Could you check a few things on this model? Use its own coordinates, in mm. A direction names the side the tool comes from. Coordinates: 2 decimals unless noted, no trailing zeros. Loops run counter-clockwise (first coordinate to the right, second up) from the corner with the lowest first, then second, coordinate; pieces in that order, holes last. Notation, with made-up numbers: (-24, 55.25) - (34, 55.25) arc R26 ccw to (34, 78.25) - close; hole circle Ø5 at (-9.5, 23.5). An arc over 180 degrees is marked (long way). One line per question, with ' | ' between items. Start each with the question number.
1. Which directions (+Z, -Z, +X, -X, +Y, -Y) give clear straight access to the entire face, cutting with the end or side of a thin tool? Please do faces 1 (the cylindrical face through (-0.116, -88.438, 49.823)), 2 (the flat face through (1.412, -89, 14)), 3 (the flat face through (-17, -89, -24.929)).
2. I want a section at C-C, the plane y = -95. Write out the boundary of the cut face in (x, z).
3. I want a section at D-D, the plane x = 41. Write out the boundary of the cut face in (y, z), then the cut area to 4 significant figures.
4. I want a section at A-A, the plane x = -57. Write out the boundary of the cut face in (y, z).
5. I'm going to push flat-ended pins straight in: P1, Ø1.5, axis at y = -73.5, z = 4, coming from the +X side; P2, Ø1, axis at y = -60, z = -44.5, coming from the +X side; P3, Ø1.5, axis at x = -22.5, z = -50.5, coming from the -Y side. Where does each tip first touch, or does it pass through?
6. Please list where these lines run through material, in increasing order: L1, parallel to X at y = -71.5, z = -4; L2, parallel to Z at x = -31, y = -103; L3, parallel to Y at x = -70.5, z = -55. Write a range as [from, to].
7. I want a section at B-B, the plane z = -61. Write out the boundary of the cut face in (x, y), then the cut area to 3 significant figures.
from build123d import *

# Parameters (mm, degrees)
F0_W     = 203.2
F0_H     = 127
F1_DEPTH = 127
F3_DEPTH = 76.2
F4_SIZE2 = 101.6
F4_SIZE  = 50.8
F5_R     = 5.08
F6_R     = 15.24
F7_DEPTH = 50.8
F8_R     = 15.24
F9_DEPTH = 127


with BuildPart() as f1:
    # F0 (on Front) → F1 (new body)
    with BuildSketch(Plane.XZ):
        with Locations((1.4119390398, -12.2287340821)):
            Rectangle(F0_W, F0_H)
    extrude(amount=F1_DEPTH)

    # F2 (on face) → F3 (cut)
    with BuildSketch(Plane.XZ.offset(127)):
        Polygon((-36.6880609602, -24.9287340821), (-36.6880609602, -75.7287340821), (103.0119390398, -75.7287340821), (103.0119390398, 51.2712659179), (1.4119390398, 51.2712659179), (1.4119390398, -24.9287340821), align=None)
    extrude(amount=-F3_DEPTH, mode=Mode.SUBTRACT)

    # F4
    f4_edges = [f1.edges().sort_by_distance(p)[0] for p in [
        (103.011939, -25.4, 51.271266),
    ]]
    f4_side = f1.faces().sort_by_distance((-20.35949, -52.614286, 51.271266))[0]
    chamfer(f4_edges, length=F4_SIZE, length2=F4_SIZE2, reference=f4_side)

    # F5
    f5_edges = [f1.edges().sort_by_distance(p)[0] for p in [
        (-49.388061, -127, 51.271266),
        (-100.188061, -63.5, 51.271266),
        (1.411939, -88.9, 51.271266),
        (26.811939, -50.8, 51.271266),
        (52.211939, -25.4, 51.271266),
        (-23.988061, 0, 51.271266),
        (77.611939, -50.8, 0.471266),
        (77.611939, 0, 0.471266),
        (103.011939, -25.4, -50.328734),
        (103.011939, 0, -63.028734),
        (103.011939, -25.4, -75.728734),
        (103.011939, -50.8, -63.028734),
        (33.161939, -50.8, -75.728734),
        (1.411939, -50.8, 13.171266),
        (1.411939, -88.9, -24.928734),
        (-36.688061, -50.8, -50.328734),
        (-17.638061, -127, -24.928734),
        (-36.688061, -127, -50.328734),
        (-68.438061, -127, -75.728734),
        (-36.688061, -88.9, -75.728734),
        (-17.638061, -50.8, -24.928734),
        (-36.688061, -88.9, -24.928734),
        (-100.188061, -127, -12.228734),
        (1.411939, -127, 13.171266),
    ]]
    fillet(f5_edges, radius=F5_R)

    # F6 (on face) → F7 (cut, through all)
    with BuildSketch(Plane.XZ.offset(50.8)):
        with Locations((19.1919390398, -37.6287340821)):
            Circle(F6_R)
    extrude(amount=-F7_DEPTH, mode=Mode.SUBTRACT)

    # F8 (on face) → F9 (cut, through all)
    with BuildSketch(Plane.XY.offset(51.2712659179)):
        with Locations((-57.0080609602, -71.12)):
            Circle(F8_R)
    extrude(amount=-F9_DEPTH, mode=Mode.SUBTRACT)


solid = f1.part
Results are:
1) face 1: +Z, +X, -Y | face 2: +Z, -Z, +X, -Y | face 3: -Z, +X, -Y
2) outline: (-100.19, -75.73) - (-41.77, -75.73) arc R5.08 ccw to (-36.69, -70.65) - (-36.69, -30.01) arc R5.08 cw to (-31.61, -24.93) - (-3.67, -24.93) arc R5.08 ccw to (1.41, -19.85) - (1.41, 46.19) arc R5.08 ccw to (-3.67, 51.27) - (-95.11, 51.27) arc R5.08 ccw to (-100.19, 46.19) - close
3) outline: (-50.8, -70.65) arc R5.08 ccw to (-45.72, -75.73) - (0, -75.73) - (0, 46.19) arc R5.08 ccw to (-5.08, 51.27) - (-45.72, 51.27) arc R5.08 ccw to (-50.8, 46.19) - close | area: 6,435 mm2
4) outline: (-127, -70.65) arc R5.08 ccw to (-121.92, -75.73) - (-86.36, -75.73) - (-86.36, 51.27) - (-121.92, 51.27) arc R5.08 ccw to (-127, 46.19) - close; (-55.88, -75.73) - (0, -75.73) - (0, 46.19) arc R5.08 ccw to (-5.08, 51.27) - (-55.88, 51.27) - close
5) P1: stops at x = 1.41 | P2: stops at x = -36.69 | P3: stops at y = -50.8
6) L1: x = [-100.19, -72.24], [-41.77, 1.41] | L2: z = [-24.93, 51.27] | L3: y = [-127, -78.21], [-64.03, 0]
7) outline: (-100.19, -121.92) arc R5.08 ccw to (-95.11, -127) - (-41.77, -127) arc R5.08 ccw to (-36.69, -121.92) - (-36.69, -55.88) arc R5.08 cw to (-31.61, -50.8) - (97.93, -50.8) arc R5.08 ccw to (103.01, -45.72) - (103.01, -5.08) arc R5.08 ccw to (97.93, 0) - (-100.19, 0) - close; hole circle Ø30.48 at (-57.01, -71.12) | area: 14,400 mm2
